```python
from build123d import *

# Parameters (mm, degrees)
SKETCH1_W               = 48
SKETCH1_H               = 50
BOSS_EXTRUDE1_DEPTH     = 70
SKETCH2_W               = 10.4
SKETCH2_H               = 20.4
CUT_EXTRUDE1_DEPTH      = 45
SKETCH3_R               = 4.15
CUT_EXTRUDE2_DEPTH      = 51
CUT_EXTRUDE3_DEPTH      = 1
CUT_EXTRUDE3_DEPTH_BACK = 71
SKETCH5_W               = 48
SKETCH5_H               = 50
CUT_EXTRUDE4_DEPTH      = 35


with BuildPart() as part:
    # Sketch1 → Boss-Extrude1 (new body)
    with BuildSketch(Plane(origin=(0, 0, 0), x_dir=(1, 0, 0), z_dir=(0, 1, 0))):
        Rectangle(SKETCH1_W, SKETCH1_H)
    extrude(amount=BOSS_EXTRUDE1_DEPTH)

    # Sketch2 → Cut-Extrude1 (cut)
    with BuildSketch(Plane(origin=(24, 0, 0), x_dir=(0, 0, -1), z_dir=(1, 0, 0))):
        with Locations((-11.5, 53)):
            Rectangle(SKETCH2_W, SKETCH2_H)
        with Locations((-11.5, 17)):
            Rectangle(SKETCH2_W, SKETCH2_H)
    extrude(amount=-CUT_EXTRUDE1_DEPTH, mode=Mode.SUBTRACT)

    # Sketch3 → Cut-Extrude2 (cut, through all)
    with BuildSketch(Plane.XY.offset(25)):
        with Locations((17, 53)):
            Circle(SKETCH3_R)
        with Locations((-17, 53)):
            Circle(SKETCH3_R)
        with Locations((-17, 17)):
            Circle(SKETCH3_R)
        with Locations((17, 17)):
            Circle(SKETCH3_R)
    extrude(amount=-CUT_EXTRUDE2_DEPTH, mode=Mode.SUBTRACT)

    # Sketch4 → Cut-Extrude3 (cut, two sides)
    with BuildSketch(Plane(origin=(0, 70, 0), x_dir=(1, 0, 0), z_dir=(0, 1, 0))) as cut_extrude3_sk:
        with BuildLine():
            Line((-7, 152.660528641), (-7, 25))
            ThreePointArc((-7, 25), (0, 18), (7, 25))
            Line((7, 25), (7, 152.660528641))
            Line((7, 152.660528641), (7, 407.981585922))
            Line((7, 407.981585922), (-7, 407.981585922))
            Line((-7, 407.981585922), (-7, 152.660528641))
        make_face()
    extrude(amount=CUT_EXTRUDE3_DEPTH, mode=Mode.SUBTRACT)
    extrude(cut_extrude3_sk.sketch, amount=-CUT_EXTRUDE3_DEPTH_BACK, mode=Mode.SUBTRACT)

    # Sketch5 → Cut-Extrude4 (cut)
    with BuildSketch(Plane.XZ):
        Rectangle(SKETCH5_W, SKETCH5_H)
    extrude(amount=-CUT_EXTRUDE4_DEPTH, mode=Mode.SUBTRACT)


solid = part.part
```
Geometry check sheet. Reference: the model listing, model coordinates, mm. A direction names the side the tool comes from. Give positions to 0.01 mm unless a question says otherwise; leave off trailing zeros. Order: outer loops, then holes, each group sorted by start corner. A loop starts at its lowest first (then second) coordinate and runs counter-clockwise, first axis right, second up. Notation, with made-up numbers: (64.25, -15) - (106.25, -15) arc R22 ccw to (106.25, 21) - close; hole circle Ø6 at (36.5, -13.5). An arc over 180 degrees is marked (long way). Answer in a Markdown table with one row per item. Add a question column.
Q1. Cross-section at A-A, the plane x = 17. Enter the section's corners in (y, z).
Q2. Gauge pin test, flat ends, axial feed: pin 1 (9.5 mm diameter, centred on x = 17, y = 53, fed in from -Z); pin 2 (4.5 mm diameter, centred on y = 47, z = 10.5, fed in from +X). Record the tip position at first contact, or that the pin passes through.
Q3. Tool access check on faces 5 (the flat face through (24, 52, 0)), 6 (the flat face through (2, 53, 6.3)). Record the directions out of +Z, -Z, +X, -X, +Y, -Y that give a thin tool (end or side, any length) a straight path to the whole face; none if there is none.
Q4. Cross-section at C-C, the plane z = -21. Enter the section's corners in (x, y).
Q5. Mould release check, pull along Z, two halves, no side actions. Record for faces 1 (the flat face through (-21, 59, 12)), 2 (the flat face through (2, 53, 16.7)), 3 (the flat face through (12, 52, -25)), 4 (the cylindrical face through (16.46, 57.115, -9.131)): pulls with the +Z half, pulls with the -Z half, needs draft (parallel to the pull), parting line crosses it, or undercut.
Q6. Cross-section at D-D, the plane y = 61.5. Enter the section's corners in (x, z).
Q7. Material ranges on probe 1 along Z at (x, y) = (-10, 45.5); probe 2 along Y at (x, z) = (-6, 12); probe 3 along X at (y, z) = (56, -7.5), recorded low to high. Write a range as from..to.
Q8. Cross-section at B-B, the plane z = 14. Enter the section's corners in (x, y), then the cut area to 3 significant figures.
Check values:
| question | item | result |
|---|---|---|
| 1 | outline | (35, -25) - (48.85, -25) - (48.85, 6.3) - (42.8, 6.3) - (42.8, 16.7) - (48.85, 16.7) - (48.85, 25) - (35, 25) - close; (57.15, -25) - (70, -25) - (70, 25) - (57.15, 25) - (57.15, 16.7) - (63.2, 16.7) - (63.2, 6.3) - (57.15, 6.3) - close |
| 2 | pin 1 | stops at z = -25 |
| 2 | pin 2 | stops at x = -21 |
| 3 | face 5 | +Z, -Z, +X, +Y, -Y |
| 3 | face 6 | +X |
| 4 | outline | (-24, 35) - (-5.74, 35) - (-5.74, 70) - (-24, 70) - close; (5.74, 35) - (24, 35) - (24, 70) - (5.74, 70) - close; hole circle Ø8.3 at (-17, 53); hole circle Ø8.3 at (17, 53) |
| 5 | face 1 | undercut |
| 5 | face 2 | undercut |
| 5 | face 3 | pulls with the -Z half |
| 5 | face 4 | needs draft |
| 6 | outline | (-24, -25) - (-7, -25) arc R7 cw to (7, -25) - (24, -25) - (24, 6.3) - (-21, 6.3) - (-21, 16.7) - (24, 16.7) - (24, 25) - (-24, 25) - close |
| 7 | probe 1 | z = -25..6.3, 16.7..25 |
| 7 | probe 2 | y = 35..42.8, 63.2..70 |
| 7 | probe 3 | x = -24..-19.87, -14.13..14.13, 19.87..24 |
| 8 | outline | (-24, 35) - (24, 35) - (24, 42.8) - (-21, 42.8) - (-21, 51.89) arc R4.15 cw to (-21, 54.11) - (-21, 63.2) - (24, 63.2) - (24, 70) - (-24, 70) - close |
| 8 | area | 762 mm^2 |
